Check sheet for the modelled part. Datum: model origin and axes. Units: mm. A direction names the side the tool comes from. Round coordinates to 2 decimals unless told otherwise and drop trailing zeros. Loops run counter-clockwise (first coordinate to the right, second up) from the corner with the lowest first, then second, coordinate; pieces in that order, holes last. Notation, with made-up numbers: (77.5, -1) -> (92.5, -1) arc R32 ccw to (92.5, 31) -> close; hole circle Ø4 at (69, -10). An arc over 180 degrees is marked (long way). Use one line per item in the form item = value. Start each with the question number.
(1) Sectioned sample at C-C (z = 11). Record the cut outline in (x, y) (3 decimals).
(2) Go/stop test with flat-tipped pins: pin 1 (3.5 mm diameter, centred on y = 4.76, z = 57.15, fed in from -X); pin 2 (5 mm diameter, centred on y = 6, z = 32, fed in from -X); pin 3 (5 mm diameter, centred on x = 9, y = 4.5, fed in from -Z); pin 4 (2.5 mm diameter, centred on y = 4.76, z = 19.05, fed in from +X). Record where each tip stops, or that it passes through.
(3) Sectioned sample at A-A (z = 101.6). Record the cut outline in (x, y) (3 decimals), and give its area (3 significant figures).
(4) Draft check along Y on faces 1 (the cylindrical face through (6.86, 4.83, 123.22)), 2 (the conical face through (35.402, 5.078, 19.149)), 3 (the flat face through (30, 0, 67)). Enter one of: released by +Y, released by -Y, zero draft, split by the parting line, or undercut.
(5) Material ranges on probe 1 along Y at (x, z) = (20.75, 57.15) (1 decimal); probe 2 along Z at (x, y) = (43, 4.5); probe 3 along Z at (x, y) = (12.5, 6), recorded low to high. Write a range as [from, to].
(6) Set-up check for faces 4 (the cylindrical face through (1.811, 4.829, 129.688)), 5 (the flat face through (9, 5, 71.603)), 6 (the cylindrical face through (17.4, 4.3, 17.2)): record each of +Z, -Z, +X, -X, +Y, -Y from which the full face is reachable in a straight line by a thin tool's end or side.
(7) Sectioned sample at B-B (y = 8.25). Record the cut outline in (x, z).
from build123d import *

# Parameters (mm, degrees)
F0_W      = 59.9948
F0_H      = 131.5974
F1_DEPTH  = 9.525
F4_D      = 4
F2_W      = 10.9474
F2_H      = 71.6026
F5_DEPTH  = 9.526
F6_R      = 6.35
F8_D      = 38.1
F10_D     = 3.81
F10_DEPTH = 12.7
F10_TIP   = 1.1446394792
F12_D     = 3.81
F12_DEPTH = 12.7
F12_TIP   = 1.1446394792


with BuildPart() as f1:
    # F0 (on Front) → F1 (new body)
    with BuildSketch(Plane.XZ):
        with Locations((29.9974, 65.7987)):
            Rectangle(F0_W, F0_H)
    extrude(amount=-F1_DEPTH)

    # F4 (through all)
    with Locations(Plane.XZ):
        with Locations((6.4262, 125.1712), (6.4262, 78.0288), (53.5686, 78.0288), (53.5686, 125.1712)):
            Hole(F4_D / 2)

    # F2 (on face) → F5 (cut, through all)
    with BuildSketch(Plane.XZ):
        with Locations((5.4737, 35.8013)):
            Rectangle(F2_W, F2_H)
        with Locations((54.5211, 35.8013)):
            Rectangle(F2_W, F2_H)
    extrude(amount=-F5_DEPTH, mode=Mode.SUBTRACT)

    # F6
    f6_edges = [f1.edges().sort_by_distance(p)[0] for p in [
        (0, 4.7625, 131.5974),
        (59.9948, 4.7625, 131.5974),
        (0, 4.7625, 71.6026),
        (59.9948, 4.7625, 71.6026),
    ]]
    fillet(f6_edges, radius=F6_R)

    # F8 (through all)
    with Locations(Plane.XZ):
        with Locations((29.9974, 101.6)):
            Hole(F8_D / 2)

    # F10
    with Locations(Plane.YZ.offset(49.0474)):
        with Locations((4.7625, 57.15), (4.7625, 19.05)):
            Hole(F10_D / 2, depth=F10_DEPTH)
            with Locations((0, 0, -(F10_DEPTH + F10_TIP / 2))):  # 118° drill point
                Cone(0, F10_D / 2, F10_TIP, mode=Mode.SUBTRACT)

    # F12
    with Locations(Plane(origin=(10.9474, 0, 0), x_dir=(0, -1, 0), z_dir=(-1, 0, 0))):
        with Locations((-4.7625, 57.15), (-4.7625, 19.05)):
            Hole(F12_D / 2, depth=F12_DEPTH)
            with Locations((0, 0, -(F12_DEPTH + F12_TIP / 2))):  # 118° drill point
                Cone(0, F12_D / 2, F12_TIP, mode=Mode.SUBTRACT)


solid = f1.part
Checks:
q1.outline = (10.947, 0) -> (49.047, 0) -> (49.047, 9.525) -> (10.947, 9.525) -> close
q2.pin_1 = 23.74
q2.pin_2 = 10.95
q2.pin_3 = 0
q2.pin_4 = 35.96
q3.outline = (0, 0) -> (10.947, 0) -> (10.947, 9.525) -> (0, 9.525) -> close; (49.047, 0) -> (59.995, 0) -> (59.995, 9.525) -> (49.047, 9.525) -> close
q3.area = 209 mm2
q4.face_1 = zero draft
q4.face_2 = undercut
q4.face_3 = released by -Y
q5.probe_1 = [0, 2.9], [6.7, 9.5]
q5.probe_2 = [0, 17.16], [20.94, 55.26], [59.04, 87.68], [115.52, 131.6]
q5.probe_3 = [0, 17.6], [20.5, 55.7], [58.6, 94.07], [109.13, 131.6]
q6.face_4 = +Z, -X, +Y, -Y
q6.face_5 = -Z, -X, +Y, -Y
q6.face_6 = -X
q7.outline = (0, 77.95) arc R6.35 ccw to (6.35, 71.6) -> (10.95, 71.6) -> (10.95, 0) -> (49.05, 0) -> (49.05, 71.6) -> (53.64, 71.6) arc R6.35 ccw to (59.99, 77.95) -> (59.99, 125.25) arc R6.35 ccw to (53.64, 131.6) -> (6.35, 131.6) arc R6.35 ccw to (0, 125.25) -> close; hole circle Ø4 at (6.43, 78.03); hole circle Ø4 at (6.43, 125.17); hole circle Ø38.1 at (30, 101.6); hole circle Ø4 at (53.57, 78.03); hole circle Ø4 at (53.57, 125.17)
